Model file for the job. Use its own axes, mm. Face numbers are marked on the shaded views. A direction names the side the tool comes from. Coordinates: 2 decimals unless noted, no trailing zeros. Write each loop counter-clockwise with the first axis right and the second up, starting at its lowest first coordinate (ties: lowest second). Pieces come first, ordered by that corner, then holes. Notation, with made-up numbers: M 20.25,11.25 L 50.25,11.25 A27 ccw 50.25,39.25 Z; hole C -34.75,14 d3. An arc over 180 degrees is marked long. Answer in a Markdown table with one row per item. Add a question column.
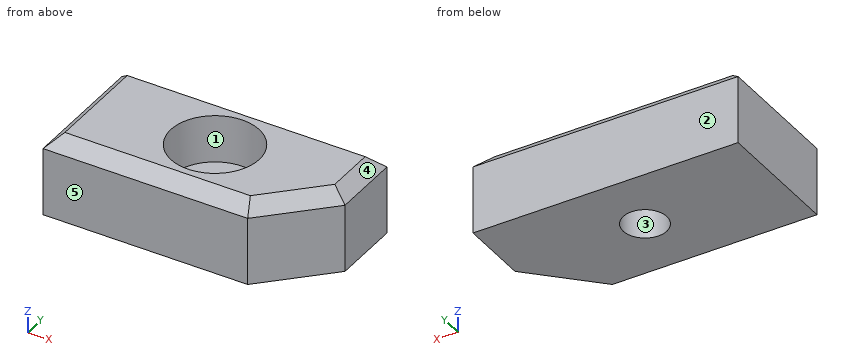
Autodesk Inventor part; units mm, degrees
ref_plane "YZ Plane" through (0, 0, 0) normal (1, 0, 0) x (0, 1, 0)
ref_plane "XZ Plane" through (0, 0, 0) normal (0, 1, 0) x (-1, 0, 0)
ref_plane "XY Plane" through (0, 0, 0) normal (0, 0, 1) x (1, 0, 0)
sketch "Эскиз1" plane through (0, 0, 0) normal (0, 0, 1) x (1, 0, 0)
  line L0 (10, 5) -> (10, -0.4101)
  line L1 (-10, 5) -> (10, 5)
  line L2 (-10, -5) -> (-10, 5)
  line L3 (5.4101, -5) -> (-10, -5)
  line L4 (10, -0.4101) -> (5.4101, -5)
  line L5 (9.75, -0.3065) -> (9.75, 4.75)
  line L6 (9.75, 4.75) -> (-9.75, 4.75)
  line L7 (-9.75, 4.75) -> (-9.75, -4.75)
  line L8 (-9.75, -4.75) -> (5.3065, -4.75)
  line L9 (5.3065, -4.75) -> (9.75, -0.3065)
  circle A0 centre (0, 0) radius 1.6
  line L10 (10, 5) -> (10, -0.4101)
  line L11 (-10, 5) -> (10, 5)
  line L12 (-10, -5) -> (-10, 5)
  line L13 (5.4101, -5) -> (-10, -5)
  line L14 (10, -0.4101) -> (5.4101, -5)
  circle A1 centre (0, 0) radius 1.6
  dimension "d0" = 0.25
extrude "Выдавливание1" add sketch "Эскиз1" along normal blind 6 contours L9 L8 L7 L6 L5
chamfer "Фаска1" distance 1 angle 45 5 edges at (-2.2218, -4.75, 6) (7.5282, -2.5282, 6) (9.75, 2.2218, 6) (0, 4.75, 6) (-9.75, 0, 6)
sketch "Эскиз2" plane through (0, 0, 6) normal (0, 0, 1) x (1, 0, 0)
  circle A0 centre (0, 0) radius 3.25
  dimension "d6" = 6.5
extrude "Выдавливание2" cut sketch "Эскиз2" against normal blind 3.5
properties part number "leg2"
1) Slice it at D-D (y = 4). Give the cut face in (x, z).
2) Which spindle directions (+Z, -Z, +X, -X, +Y, -Y) get a long thin tool onto all of the face, cutting with end or side? Do the marked faces 1 and 2. Say none if no direction does.
3) Two-plate mould, pull along Y, no slides. Class the marked faces 3, 4 and 5: released by +Y, released by -Y, zero draft, split by the parting line, or undercut.
4) Slice it at A-A (x = 0). Give the cut face in (y, z).
5) Drill centre lines: probe 1 along Y at (x, z) = (0, 3.4); probe 2 along X at (y, z) = (0, 1); probe 3 along Y at (x, z) = (0, 1.15). Where is each one in solid material? Low to high.
6) Slice it at C-C (y = 0.5). Give the cut face in (x, z), then the cut area to 3 significant figures.
7) Slice it at B-B (z = 3.25). Give the cut face in (x, y).
Ans:
| question | item | result |
|---|---|---|
| 1 | outline | M -9.75,0 L 9.75,0 L 9.75,5 L 9,5.75 L -9,5.75 L -9.75,5 Z |
| 2 | face 1 | +Z |
| 2 | face 2 | +Z, -Z, +X, -X, +Y |
| 3 | face 3 | undercut |
| 3 | face 4 | zero draft |
| 3 | face 5 | released by -Y |
| 4 | outline | M -4.75,0 L -1.6,0 L -1.6,2.5 L -3.25,2.5 L -3.25,6 L -3.75,6 L -4.75,5 Z; M 1.6,0 L 4.75,0 L 4.75,5 L 3.75,6 L 3.25,6 L 3.25,2.5 L 1.6,2.5 Z |
| 5 | probe 1 | y = -4.75 to -3.25, 3.25 to 4.75 |
| 5 | probe 2 | x = -9.75 to -1.6, 1.6 to 9.75 |
| 5 | probe 3 | y = -4.75 to -1.6, 1.6 to 4.75 |
| 6 | outline | M -9.75,0 L -1.52,0 L -1.52,2.5 L -3.21,2.5 L -3.21,6 L -8.75,6 L -9.75,5 Z; M 1.52,0 L 9.75,0 L 9.75,5 L 8.75,6 L 3.21,6 L 3.21,2.5 L 1.52,2.5 Z |
| 6 | area | 85.9 mm2 |
| 7 | outline | M -9.75,-4.75 L 5.31,-4.75 L 9.75,-0.31 L 9.75,4.75 L -9.75,4.75 Z; hole C 0,0 d6.5 |
